Check sheet for the drawn part. Datum: minimum x, y, z corner. Units: mm. Coordinates: 2 decimals unless noted, no trailing zeros. Order: outer loops, then holes, each group sorted by start corner. A loop starts at its lowest first (then second) coordinate and runs counter-clockwise, first axis right, second up.
Q1. Thickness scan on line 1 (Z direction, x = 21, y = 12.5); line 2 (X direction, y = 19.5, z = 58); line 3 (Y direction, x = 10.5, z = 59). Record the ranges inside material, lowest first.
Q2. Draft check along Z on the marked faces 1, 2, 3 and 4. Enter one of: pulls with the +Z half, pulls with the -Z half, needs draft (parallel to the pull), parting line crosses it, or undercut.
Q3. Depth check by flat-ended pin: P1, Ø11.5, axis at x = 15.5, z = 62, coming from the +Y side; P2, Ø2, axis at x = 14, y = 7, coming from the -Z side. Enter the tip coordinate at first touch or a pass-through.
Q4. Cross-section at C-C, the plane z = 58. Record the boundary of the cut face in (x, y).
Q5. Cross-section at B-B, the plane x = 8.5. Record the boundary of the cut face in (y, z).
Q6. Cross-section at A-A, the plane y = 12.75. Record the boundary of the cut face in (x, z), and give its area (3 significant figures).
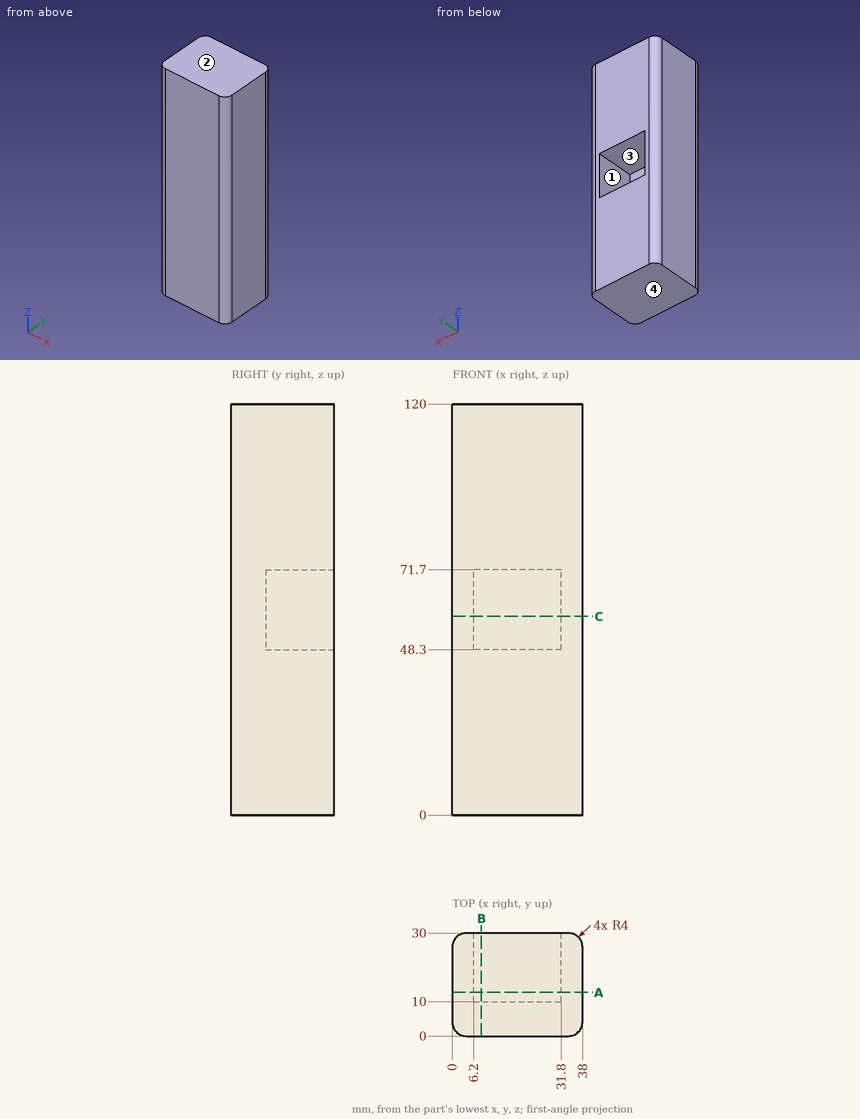
Check values:
1. line 1: z = 0 to 48.3, 71.7 to 120
1. line 2: x = 0 to 6.2, 31.8 to 38
1. line 3: y = 0 to 10
2. face 1: undercut
2. face 2: pulls with the +Z half
2. face 3: undercut
2. face 4: pulls with the -Z half
3. P1: stops at y = 10
3. P2: stops at z = 0
4. outline: (0, 4) arc R4 ccw to (4, 0) - (34, 0) arc R4 ccw to (38, 4) - (38, 26) arc R4 ccw to (34, 30) - (31.8, 30) - (31.8, 10) - (6.2, 10) - (6.2, 30) - (4, 30) arc R4 ccw to (0, 26) - close
5. outline: (0, 0) - (30, 0) - (30, 48.3) - (10, 48.3) - (10, 71.7) - (30, 71.7) - (30, 120) - (0, 120) - close
6. outline: (0, 0) - (38, 0) - (38, 120) - (0, 120) - close; hole (6.2, 48.3) - (31.8, 48.3) - (31.8, 71.7) - (6.2, 71.7) - close
6. area: 3,960 mm2
